Design review of the part shown in the three views and the two pictorial views. Dimensions are in mm from the part's minimum x, y and z. A direction names the side the tool comes from. Coordinates: 2 decimals unless noted, no trailing zeros. Loops run counter-clockwise (first coordinate to the right, second up) from the corner with the lowest first, then second, coordinate; pieces in that order, holes last. Notation, with made-up numbers: (37, 63.25) -> (82, 63.25) arc R18 ccw to (82, 67.25) -> close; hole circle Ø9 at (57, 88). An arc over 180 degrees is marked (long way). One line per item, written item: value. Start each with the question number.
1. Add section D-D on z = 31. Write out the cut boundary in (x, y).
2. Add section B-B on y = 20. Write out the cut boundary in (x, z) (1 decimal), plus the area to 3 significant figures.
3. For probe 1 along Y at (x, z) = (1.25, 63.25); probe 2 along X at (y, z) = (10, 17); probe 3 along Z at (x, y) = (5, 21.5), list the stretches that pass through material, from the lowest coordinate up.
4. Insertion check: pin 1 (7.5 mm diameter, centred on y = 20.93, z = 63.25, fed in from +X); pin 2 (4 mm diameter, centred on x = 15, y = 33.5, fed in from -Z); pin 3 (8 mm diameter, centred on x = 23.5, y = 12.5, fed in from -Z). Each pin has a flat end and moves straight along its axis. Give the tip position at first contact, or say it passes through.
5. Add section C-C on y = 3. Write out the cut boundary in (x, z), plus the area to 3 significant figures.
6. Machinability: for the marked faces 1 and 2, which of the approach directions +Z, -Z, +X, -X, +Y, -Y give a long, thin tool a straight path to every point of the face, cutting with its end or side? Answer none if there is none.
7. Add section A-A on z = 6.75. Write out the cut boundary in (x, y).
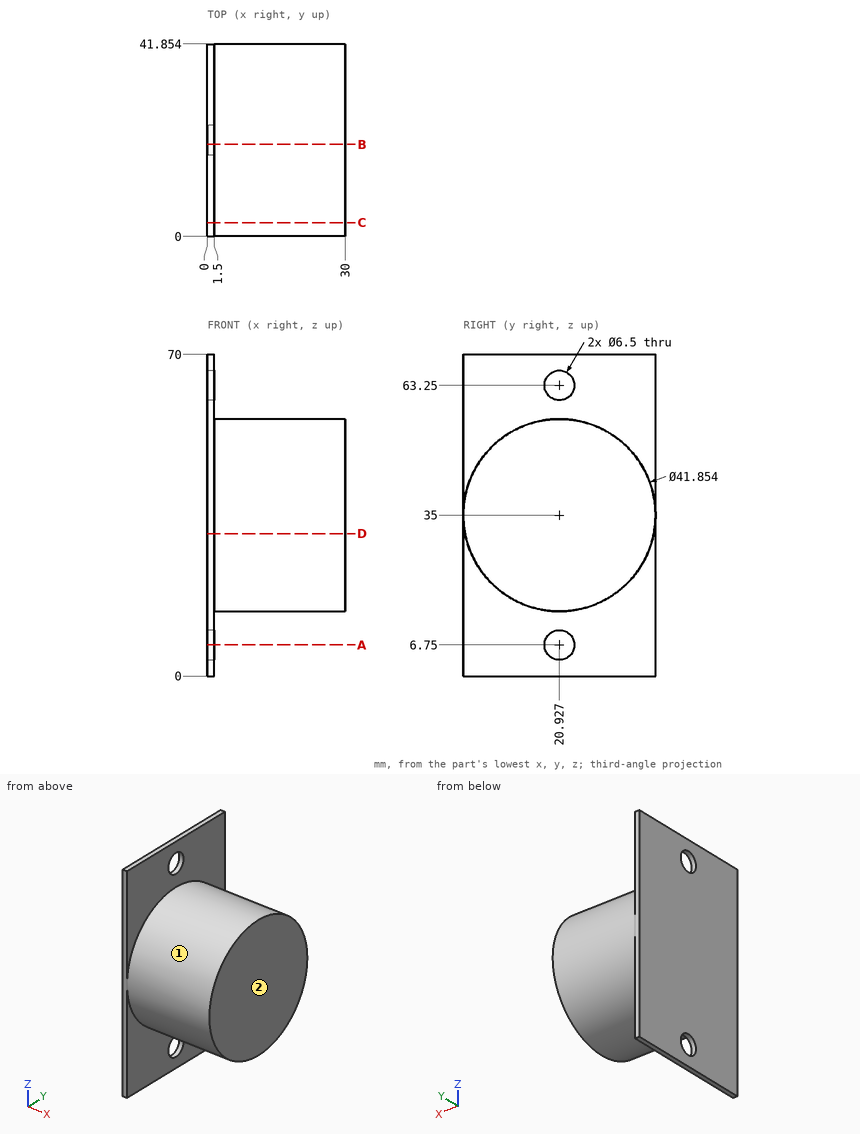
Worked answers:
1. outline: (0, 0) -> (1.5, 0) -> (1.5, 0.39) -> (30, 0.39) -> (30, 41.47) -> (1.5, 41.47) -> (1.5, 41.85) -> (0, 41.85) -> close
2. outline: (0, 0) -> (1.5, 0) -> (1.5, 3.6) -> (0, 3.6) -> close; (0, 9.9) -> (1.5, 9.9) -> (1.5, 14.1) -> (30, 14.1) -> (30, 55.9) -> (1.5, 55.9) -> (1.5, 60.1) -> (0, 60.1) -> close; (0, 66.4) -> (1.5, 66.4) -> (1.5, 70) -> (0, 70) -> close
2. area: 1,280 mm²
3. probe 1: y = 0 to 17.68, 24.18 to 41.85
3. probe 2: x = 0 to 1.5
3. probe 3: z = 14.08 to 55.92
4. pin 1: stops at x = 1.5
4. pin 2: stops at z = 16.94
4. pin 3: stops at z = 14.55
5. outline: (0, 0) -> (1.5, 0) -> (1.5, 24.2) -> (30, 24.2) -> (30, 45.8) -> (1.5, 45.8) -> (1.5, 70) -> (0, 70) -> close
5. area: 720 mm²
6. face 1: +X
6. face 2: +Z, -Z, +X, +Y, -Y
7. outline: (0, 0) -> (1.5, 0) -> (1.5, 17.68) -> (0, 17.68) -> close; (0, 24.18) -> (1.5, 24.18) -> (1.5, 41.85) -> (0, 41.85) -> close
